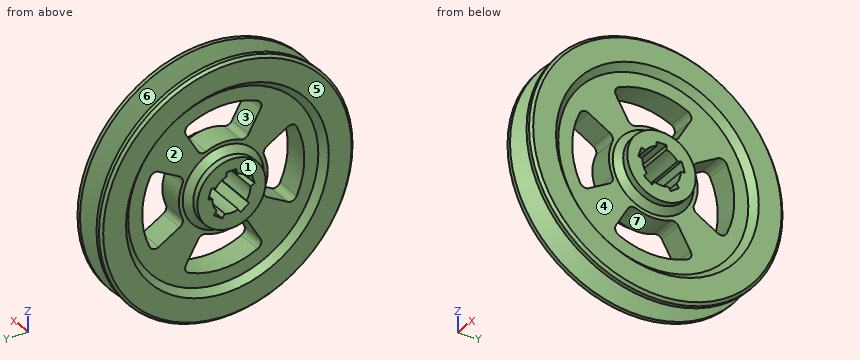
from build123d import *

# Parameters (mm, degrees)
F3_DEPTH = 70


with BuildPart() as f1:
    # F0 (on Top) → F1 (revolve)
    with BuildSketch(Plane.XY):
        Polygon((20, -27), (20, 0), (-20, 0), (-20, -27), (-15, -27), (-10, -32), (-10, -75), (-15, -80), (-15, -98), (-13, -100), (-10, -100), (-4.641016, -80), (0, -80), (4.641016, -80), (10, -100), (13, -100), (15, -98), (15, -80), (10, -75), (10, -32), (15, -27), align=None)
    revolve(axis=Axis((0, 0, 0), (1, 0, 0)))

    # F2 (on face) → F3 (cut, symmetric)
    with BuildSketch(Plane.YZ.offset(10)):
        with BuildLine():
            ThreePointArc((29.393877, 50.911688), (29.83415, 54.909449), (27.187796, 57.938103))
            ThreePointArc((27.187796, 57.938103), (0, 64), (-27.187796, 57.938103))
            ThreePointArc((-27.187796, 57.938103), (-29.83415, 54.909449), (-29.393877, 50.911688))
            Line((-29.393877, 50.911688), (-19.843135, 34.369318))
            ThreePointArc((-19.843135, 34.369318), (-17.107009, 32.130208), (-13.573882, 32.260653))
            ThreePointArc((-13.573882, 32.260653), (0, 35), (13.573882, 32.260653))
            ThreePointArc((13.573882, 32.260653), (17.107009, 32.130208), (19.843135, 34.369318))
            Line((19.843135, 34.369318), (29.393877, 50.911688))
        make_face()
        with BuildLine():
            Line((-4, 18), (-4, 14.456832))
            ThreePointArc((-4, 14.456832), (-8.816779, 12.135255), (-12.513197, 8.271633))
            Line((-12.513197, 8.271633), (-15.882949, 9.366532))
            Line((-15.882949, 9.366532), (-18.355085, 1.75808))
            Line((-18.355085, 1.75808), (-14.985333, 0.663181))
            ThreePointArc((-14.985333, 0.663181), (-14.265848, -4.635255), (-11.733581, -9.344682))
            Line((-11.733581, -9.344682), (-13.816203, -12.211165))
            Line((-13.816203, -12.211165), (-7.344067, -16.913447))
            Line((-7.344067, -16.913447), (-5.261445, -14.046964))
            ThreePointArc((-5.261445, -14.046964), (0, -15), (5.261445, -14.046964))
            Line((5.261445, -14.046964), (7.344067, -16.913447))
            Line((7.344067, -16.913447), (13.816203, -12.211165))
            Line((13.816203, -12.211165), (11.733581, -9.344682))
            ThreePointArc((11.733581, -9.344682), (14.265848, -4.635255), (14.985333, 0.663181))
            Line((14.985333, 0.663181), (18.355085, 1.75808))
            Line((18.355085, 1.75808), (15.882949, 9.366532))
            Line((15.882949, 9.366532), (12.513197, 8.271633))
            ThreePointArc((12.513197, 8.271633), (8.816779, 12.135255), (4, 14.456832))
            Line((4, 14.456832), (4, 18))
            Line((4, 18), (-4, 18))
        make_face()
        with BuildLine():
            ThreePointArc((-50.911688, 29.393877), (-54.909449, 29.83415), (-57.938103, 27.187796))
            ThreePointArc((-57.938103, 27.187796), (-64, 0), (-57.938103, -27.187796))
            ThreePointArc((-57.938103, -27.187796), (-54.909449, -29.83415), (-50.911688, -29.393877))
            Line((-50.911688, -29.393877), (-34.369318, -19.843135))
            ThreePointArc((-34.369318, -19.843135), (-32.130208, -17.107009), (-32.260653, -13.573882))
            ThreePointArc((-32.260653, -13.573882), (-35, 0), (-32.260653, 13.573882))
            ThreePointArc((-32.260653, 13.573882), (-32.130208, 17.107009), (-34.369318, 19.843135))
            Line((-34.369318, 19.843135), (-50.911688, 29.393877))
        make_face()
        with BuildLine():
            ThreePointArc((-29.393877, -50.911688), (-29.83415, -54.909449), (-27.187796, -57.938103))
            ThreePointArc((-27.187796, -57.938103), (0, -64), (27.187796, -57.938103))
            ThreePointArc((27.187796, -57.938103), (29.83415, -54.909449), (29.393877, -50.911688))
            Line((29.393877, -50.911688), (19.843135, -34.369318))
            ThreePointArc((19.843135, -34.369318), (17.107009, -32.130208), (13.573882, -32.260653))
            ThreePointArc((13.573882, -32.260653), (0, -35), (-13.573882, -32.260653))
            ThreePointArc((-13.573882, -32.260653), (-17.107009, -32.130208), (-19.843135, -34.369318))
            Line((-19.843135, -34.369318), (-29.393877, -50.911688))
        make_face()
        with BuildLine():
            ThreePointArc((50.911688, -29.393877), (54.909449, -29.83415), (57.938103, -27.187796))
            ThreePointArc((57.938103, -27.187796), (64, 0), (57.938103, 27.187796))
            ThreePointArc((57.938103, 27.187796), (54.909449, 29.83415), (50.911688, 29.393877))
            Line((50.911688, 29.393877), (34.369318, 19.843135))
            ThreePointArc((34.369318, 19.843135), (32.130208, 17.107009), (32.260653, 13.573882))
            ThreePointArc((32.260653, 13.573882), (35, 0), (32.260653, -13.573882))
            ThreePointArc((32.260653, -13.573882), (32.130208, -17.107009), (34.369318, -19.843135))
            Line((34.369318, -19.843135), (50.911688, -29.393877))
        make_face()
    extrude(amount=F3_DEPTH, both=True, mode=Mode.SUBTRACT)


solid = f1.part
CAD build for the part. Positions are in the model's coordinates, mm. Face numbers are marked on the shaded views. A direction names the side the tool comes from. Coordinates: 2 decimals unless noted, no trailing zeros.
Item 1: Band-saw the part on A-A on y = 0. Give the number of separate pieces and of enclosed holes in the cut face, plus the area to 3 significant figures.
Check sheet entries:
separate pieces: 4
enclosed holes: 0
area: 2,510 mm2
Item 2: 3-axis set-ups, long thin cutter, end or side, ignore diameter. For the marked faces 1, 2, 3 and 4: which of +Z, -Z, +X, -X, +Y, -Y reach the whole face in a straight line?
Check sheet entries:
face 1: +Z, -Z, -X, +Y, -Y
face 2: -X
face 3: +X, -X
face 4: +X
Item 3: Two-plate mould, pull along Y, no slides. Class the marked faces 5, 6 and 7: +Y half, -Y half, draft (parallel to the pull), parting line (faces both ways), or undercut.
Check sheet entries:
face 5: draft
face 6: parting line
face 7: undercut
Item 4: Pin check, flat tips, straight feed: pin 1 Ø6 at (y, z) = (-77, -6.5) entering from -X; pin 2 Ø1.5 at (x, y) = (10.5, 35) entering from -Z; pin 3 Ø6.5 at (x, y) = (1, 1.5) entering from -Z. Stop position of each tip, or through.
Check sheet entries:
pin 1: stops at x = -15
pin 2: stops at z = -93.95
pin 3: stops at z = -80
Item 5: Drill centre lines: L1, parallel to Y at x = 14.5, z = 19.5; L2, parallel to Z at x = 13, y = 13; L3, parallel to Z at x = 2, y = 26. Where is each one in solid material? Low to high.
Check sheet entries:
L1: y = -96.55 to -77.07, -19.39 to 19.39, 77.07 to 96.55
L2: z = -99.15 to -76.91, -25.92 to -12.8, -11.09 to -7.48, 8.43 to 25.92, 76.91 to 99.15
L3: z = -75.66 to -58.48, -45.03 to 45.03, 58.48 to 75.66
